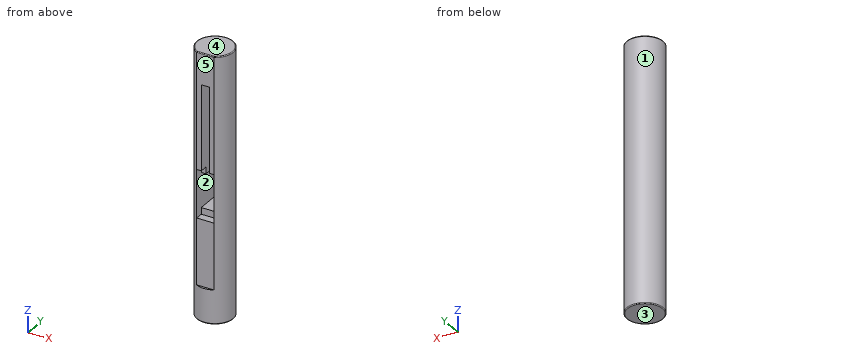
```python
from build123d import *

# Parameters (mm, degrees)
SKETCH_1_R               = 22
EXTRUDE_1_DEPTH          = 320
SKETCH_3_W               = 21
SKETCH_3_H               = 42
CUT_EXTRUDE_1_DEPTH      = 40
CUT_EXTRUDE_2_DEPTH      = 130
CUT_EXTRUDE_2_DEPTH_BACK = 150
SKETCH_8_W               = 21
SKETCH_8_H               = 8
CUT_EXTRUDE_5_DEPTH      = 9.2
SKETCH_9_W               = 9.811196784
SKETCH_9_H               = 111
CUT_EXTRUDE_6_DEPTH      = 37.332615
FILLET_1_R               = 1
FILLET_2_R               = 1


with BuildPart() as part:
    # Sketch 1 → Extrude 1 (new body)
    with BuildSketch(Plane.XY):
        Circle(SKETCH_1_R)
    extrude(amount=EXTRUDE_1_DEPTH)

    # Sketch 3 → Cut-Extrude 1 (cut)
    with BuildSketch(Plane(origin=(0, -22, 0), x_dir=(-1, 0, 0), z_dir=(0, -1, 0))):
        with Locations((0, -150)):
            Rectangle(SKETCH_3_W, SKETCH_3_H)
    extrude(amount=-CUT_EXTRUDE_1_DEPTH, mode=Mode.SUBTRACT)

    # Sketch 5 → Cut-Extrude 2 (cut, two sides)
    with BuildSketch(Plane(origin=(0, 0, 171), x_dir=(-1, 0, 0), z_dir=(0, 0, -1))) as cut_extrude_2_sk:
        with BuildLine():
            Line((10.5, -19.332614929), (-10.5, -19.332614929))
            ThreePointArc((-10.5, -19.332614929), (0, -22), (10.5, -19.332614929))
        make_face()
    extrude(amount=CUT_EXTRUDE_2_DEPTH, mode=Mode.SUBTRACT)
    extrude(cut_extrude_2_sk.sketch, amount=-CUT_EXTRUDE_2_DEPTH_BACK, mode=Mode.SUBTRACT)

    # Sketch 8 → Cut-Extrude 5 (cut)
    with BuildSketch(Plane(origin=(0, -19.332614929, 0), x_dir=(-1, 0, 0), z_dir=(0, -1, 0))):
        with Locations((0, -175)):
            Rectangle(SKETCH_8_W, SKETCH_8_H)
        with Locations((0, -125)):
            Rectangle(SKETCH_8_W, SKETCH_8_H)
    extrude(amount=-CUT_EXTRUDE_5_DEPTH, mode=Mode.SUBTRACT)

    # Sketch 9 → Cut-Extrude 6 (cut)
    with BuildSketch(Plane(origin=(0, -19.332614929, 0), x_dir=(-1, 0, 0), z_dir=(0, -1, 0))):
        with Locations((0, -226.5)):
            Rectangle(SKETCH_9_W, SKETCH_9_H)
    extrude(amount=-CUT_EXTRUDE_6_DEPTH, mode=Mode.SUBTRACT)

    # Fillet 1
    fillet_1_edges = [part.edges().sort_by_distance(p)[0] for p in [
        (-22, 0, 0),
    ]]
    fillet(fillet_1_edges, radius=FILLET_1_R)

    # Fillet 2
    fillet_2_edges = [part.edges().sort_by_distance(p)[0] for p in [
        (-11.247221879, 18.907670401, 320),
        (0, -19.332614929, 320),
    ]]
    fillet(fillet_2_edges, radius=FILLET_2_R)


solid = part.part
```
For this review, take the finished solid that the model builds, in its own axes (mm). Face numbers are marked on the shaded views. A direction names the side the tool comes from. Coordinates: 2 decimals unless noted, no trailing zeros. Write each loop counter-clockwise with the first axis right and the second up, starting at its lowest first coordinate (ties: lowest second). Pieces come first, ordered by that corner, then holes.
(1) Add section A-A on y = 0. Give the boundary of the cut face in (x, z), then the cut area to 3 significant figures.
(2) The part is to be moulded in two halves that separate along X. For the marked faces 1, 2 and 3, say which applies: +X half, -X half, draft (parallel to the pull), parting line (faces both ways), or undercut.
(3) Wall thickness on probe 1 along Z at (x, y) = (-1.5, 2); probe 2 along Z at (x, y) = (9, 5); probe 3 along X at (y, z) = (-1, 144.5): over which ranges is each line inside the solid? List them lowest first.
(4) Add section D-D on z = 175.5. Give the boundary of the cut face in (x, y), then the cut area to 3 significant figures.
(5) For pin 1 Ø6.5 at (x, z) = (-5, 124) entering from -Y; pin 2 Ø1.5 at (y, z) = (-7, 252.5) entering from -X; pin 3 Ø1.7 at (x, z) = (-7.5, 176) entering from -Y, all flat-tipped, find the tip position at first contact; note any pin that passes through.
(6) Tool access review of the marked faces 4 and 5: name each direction out of +Z, -Z, +X, -X, +Y, -Y from which nothing blocks a thin tool from reaching the whole face with its end or side.
(7) Add section B-B on x = 0. Give the boundary of the cut face in (y, z), then the cut area to 3 significant figures.
(8) Add section C-C on z = 211.5. Give the boundary of the cut face in (x, y), then the cut area to 3 significant figures.
Answer sheet:
1. outline: (-22, 1) arc R1 ccw to (-21, 0) - (21, 0) arc R1 ccw to (22, 1) - (22, 319) arc R1 ccw to (21, 320) - (-21, 320) arc R1 ccw to (-22, 319) - close; hole (-10.5, 129) - (10.5, 129) - (10.5, 171) - (4.91, 171) - (4.91, 282) - (-4.91, 282) - (-4.91, 171) - (-10.5, 171) - close
1. area: 12,100 mm2
2. face 1: parting line
2. face 2: undercut
2. face 3: draft
3. probe 1: z = 0 to 129, 282 to 320
3. probe 2: z = 0 to 129, 171 to 320
3. probe 3: x = -21.98 to -10.5, 10.5 to 21.98
4. outline: (-10.5, -19.33) - (-10.5, -10.13) - (-4.91, -10.13) - (-4.91, 18) - (4.91, 18) - (4.91, -10.13) - (10.5, -10.13) - (10.5, -19.33) arc R22 ccw (long way) to start
4. area: 1,010 mm2
5. pin 1: stops at y = -19.33
5. pin 2: stops at x = -21.09
5. pin 3: stops at y = -10.13
6. face 4: +Z, +X, -X, +Y, -Y
6. face 5: +Z, +X, -X, -Y
7. outline: (-22, 1) arc R1 ccw to (-21, 0) - (21, 0) arc R1 ccw to (22, 1) - (22, 319) arc R1 ccw to (21, 320) - (-18.33, 320) arc R1 ccw to (-19.33, 319) - (-19.33, 282) - (18, 282) - (18, 129) - (-10.13, 129) - (-10.13, 121) - (-19.33, 121) - (-19.33, 41) - (-22, 41) - close
7. area: 7,550 mm2
8. outline: (-10.5, -19.33) - (-4.91, -19.33) - (-4.91, 18) - (4.91, 18) - (4.91, -19.33) - (10.5, -19.33) arc R22 ccw (long way) to start
8. area: 1,120 mm2
